from build123d import *

# Parameters (mm, degrees)
MAIN_BLOCK_EXTRUDE_DEPTH = 65.09
SHELL1_T                 = -5


with BuildPart() as part:
    # Sketch1 → Main block extrude (new, symmetric)
    with BuildSketch(Plane(origin=(0, 0, 0), x_dir=(1, 0, 0), z_dir=(0, 1, 0))):
        Polygon((0, 0), (-71.265, -399.066716446), (71.265, -399.066716446), align=None)
    extrude(amount=MAIN_BLOCK_EXTRUDE_DEPTH, both=True)

    # Shell1
    shell1_openings = [part.faces().sort_by_distance(p)[0] for p in [
        (0, -65.09, 266.044477631),
    ]]
    offset(amount=SHELL1_T, openings=shell1_openings, kind=Kind.INTERSECTION)


solid = part.part
Geometry check sheet. Reference: the model listing, model coordinates, mm. A direction names the side the tool comes from. Coordinates: 2 decimals unless noted, no trailing zeros. Order: outer loops, then holes, each group sorted by start corner. A loop starts at its lowest first (then second) coordinate and runs counter-clockwise, first axis right, second up. Notation, with made-up numbers: (73.25, 49.25) - (95.25, 49.25) arc R17 ccw to (95.25, 78.25) - close; hole circle Ø8 at (31.25, -16). An arc over 180 degrees is marked (long way). Answer in a Markdown table with one row per item. Add a question column.
1) Gauge pin test, flat ends, axial feed: P1, Ø5, axis at x = -41, z = 318.5, coming from the -Y side; P2, Ø12, axis at y = 38.5, z = 230.5, coming from the -X side; P3, Ø6, axis at y = 40.5, z = 218.5, coming from the +X side. Record the tip position at first contact, or that the pin passes through.
2) Release check for a two-part mould opening along Z. For faces 3 (the flat face through (-1, 60.09, 249)), 4 (the flat face through (-1, 1, 399.067)), 5 (the flat face through (31, -65.09, 199)) record: +Z half, -Z half, draft (parallel to the pull), parting line (faces both ways), or undercut.
3) Cross-section at C-C, the plane z = 243.5. Record the cut outline in (x, y), then the cut area to 3 significant figures.
4) Set-up check for faces 1 (the flat face through (33.1, -1.6, 213.8)), 2 (the flat face through (-35.134, 0.911, 196.74)): record each of +Z, -Z, +X, -X, +Y, -Y from which the full face is reachable in a straight line by a thin tool's end or side.
5) Cross-section at A-A, the plane y = -52.5. Record the cut outline in (x, z) (3 decimals).
6) Material ranges on line 1 along X through (y, z) = (-40.5, 355.5); line 2 along X through (y, z) = (40, 380.5); line 3 along Y through (x, z) = (21, 363.5), recorded low to high. Write a range as [from, to].
7) Cross-section at B-B, the plane x = 26. Record the cut outline in (y, z), then the cut area to 3 significant figures.
Check result:
| question | item | result |
|---|---|---|
| 1 | P1 | stops at y = 60.09 |
| 1 | P2 | stops at x = -42.23 |
| 1 | P3 | stops at x = 39.56 |
| 2 | face 3 | undercut |
| 2 | face 4 | +Z half |
| 2 | face 5 | draft |
| 3 | outline | (-43.48, -65.09) - (-38.4, -65.09) - (-38.4, 60.09) - (38.4, 60.09) - (38.4, -65.09) - (43.48, -65.09) - (43.48, 65.09) - (-43.48, 65.09) - close |
| 3 | area | 1,710 mm² |
| 4 | face 1 | -Y |
| 4 | face 2 | -Z, -X, +Y, -Y |
| 5 | outline | (-71.265, 399.067) - (0, 0) - (71.265, 399.067) - close; hole (-65.293, 394.067) - (0, 28.442) - (65.293, 394.067) - close |
| 6 | line 1 | x = [-63.48, -58.41], [58.41, 63.48] |
| 6 | line 2 | x = [-67.95, -62.87], [62.87, 67.95] |
| 6 | line 3 | y = [60.09, 65.09] |
| 7 | outline | (-65.09, 145.59) - (65.09, 145.59) - (65.09, 399.07) - (-65.09, 399.07) - (-65.09, 394.07) - (60.09, 394.07) - (60.09, 174.04) - (-65.09, 174.04) - close |
| 7 | area | 5,450 mm² |
